Verification items for the finished model (mm, model axes). Round coordinates to 2 decimals unless told otherwise and drop trailing zeros. Order: outer loops, then holes, each group sorted by start corner. A loop starts at its lowest first (then second) coordinate and runs counter-clockwise, first axis right, second up. Notation, with made-up numbers: (-28.5, 61) -> (-19.5, 61) arc R16 ccw to (-19.5, 67) -> close; hole circle Ø10 at (27.25, 24). An arc over 180 degrees is marked (long way). Put each result on its own line as item: value.
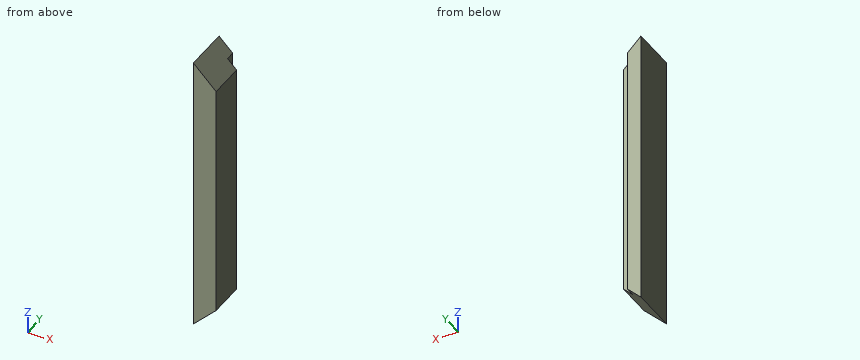
from build123d import *

# Parameters (mm, degrees)
F1_DEPTH = 196.85
F3_DEPTH = 31.751


with BuildPart() as f1:
    # F0 (on Top) → F1 (new body)
    with BuildSketch(Plane.XY):
        Polygon((1.5875, 9.525), (1.5875, 15.875), (-7.9375, 15.875), (-7.9375, -15.875), (7.9375, -15.875), (7.9375, 9.525), align=None)
    extrude(amount=F1_DEPTH)

    # F2 (on face) → F3 (cut, through all)
    with BuildSketch(Plane.XZ.offset(15.875)):
        Polygon((7.9375, 196.85), (-7.9375, 196.85), (7.9375, 180.975), align=None)
        Polygon((7.9375, 15.875), (-7.9375, 0), (7.9375, 0), align=None)
    extrude(amount=-F3_DEPTH, mode=Mode.SUBTRACT)


solid = f1.part
Item 1: Gauge pin test, flat ends, axial feed: pin 1 Ø4 at (x, y) = (-4.5, 3.5) entering from +Z; pin 2 Ø1.9 at (x, z) = (4.5, 126) entering from +Y (3 decimals); pin 3 Ø8 at (x, y) = (1.5, -11.5) entering from +Z. Record the tip position at first contact, or that the pin passes through.
Check sheet entries:
pin 1: stops at z = 195.41
pin 2: stops at y = 9.525
pin 3: stops at z = 191.41
Item 2: Section check A-A on z = 71. Record the boundary of the cut face in (x, y) (1 decimal).
Check sheet entries:
outline: (-7.9, -15.9) -> (7.9, -15.9) -> (7.9, 9.5) -> (1.6, 9.5) -> (1.6, 15.9) -> (-7.9, 15.9) -> close
Item 3: Section check C-C on x = 6. Record the boundary of the cut face in (y, z) (1 decimal), then the cut area to 3 significant figures.
Check sheet entries:
outline: (-15.9, 13.9) -> (9.5, 13.9) -> (9.5, 182.9) -> (-15.9, 182.9) -> close
area: 4,290 mm^2
Item 4: Material ranges on L1, parallel to Y at x = 6, z = 74.5 (3 decimals); L2, parallel to X at y = 15, z = 148.5; L3, parallel to Z at x = -6, y = 7, recorded low to high. Write a range as [from, to].
Check sheet entries:
L1: y = [-15.875, 9.525]
L2: x = [-7.94, 1.59]
L3: z = [1.94, 194.91]
